Source: three-view drawing plus pictorial views. Frame: mm from the lowest corner of the part. A direction names the side the tool comes from. Give positions to 0.01 mm unless a question says otherwise; leave off trailing zeros. Loops run counter-clockwise (first coordinate to the right, second up) from the corner with the lowest first, then second, coordinate; pieces in that order, holes last. Notation, with made-up numbers: M -5,-6.75 L 33,-6.75 A12 cw 33,3.25 Z; hole C 30,71.25 d5. An arc over 180 degrees is marked long. Answer as a JSON object with one key per item and string values. Group by question number.
1) Ray query, L1, parallel to Y at x = 20, z = 12; L2, parallel to X at y = 20, z = 13; L3, parallel to X at y = 12, z = 13.5. Return the intervals inside material, ascending.
2) Access query for the marked faces 1 and 2. Directions: +Z, -Z, +X, -X, +Y, -Y. A direction counts if a zero-diameter tool reaches every point of the face in a straight line with its end or side. Return the directions, or none.
3) Draft query along Y for the marked faces 3, 4 and 5. Return one class per face: +Y half, -Y half, draft (parallel to the pull), parting line (faces both ways), or undercut.
4) Section query B-B on z = 12.5. Return loops of the section in (x, y), plus the area to 3 significant figures.
5) Section query D-D on x = 49. Return loops of the section in (y, z).
6) Section query A-A on x = 20. Return loops of the section in (y, z), plus the area to 3 significant figures.
7) First-contact query: P1, Ø5, axis at x = 4, z = 27, coming from the +Y side; P2, Ø1.5, axis at x = 32.5, z = 8.5, coming from the +Y side; P3, Ø6, axis at x = 36, y = 32, coming from the +Z side. Flat tips, straight axial feed; report the tip coordinate or a pass-through.
8) Section query C-C on y = 14.5. Return loops of the section in (x, z), plus the area to 3 significant figures.
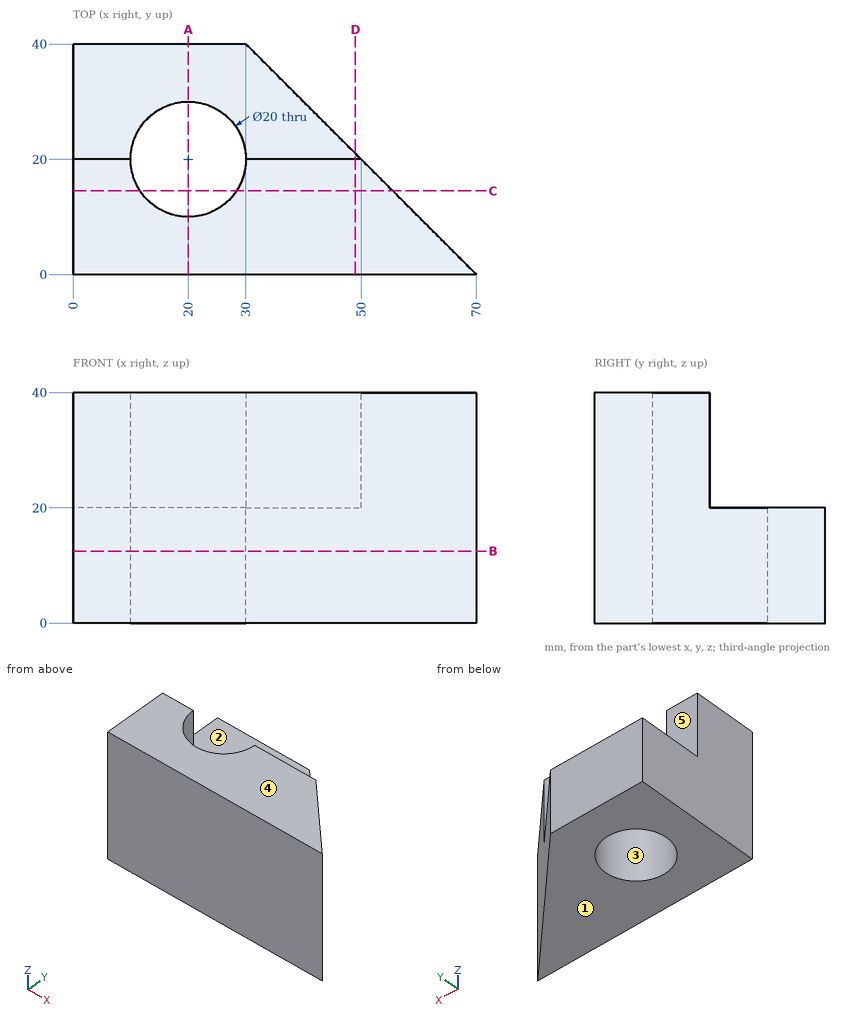
Output:
{
 "1": {"L1": "y = 0 to 10, 30 to 40", "L2": "x = 0 to 10, 30 to 50", "L3": "x = 0 to 14, 26 to 58"},
 "2": {"face 1": "-Z, +X, -X, +Y, -Y", "face 2": "+Z, +X, -X, +Y"},
 "3": {"face 3": "undercut", "face 4": "draft", "face 5": "+Y half"},
 "4": {"outline": "M 0,0 L 70,0 L 30,40 L 0,40 Z; hole C 20,20 d20", "area": "1,690 mm^2"},
 "5": {"outline": "M 0,0 L 21,0 L 21,20 L 20,20 L 20,40 L 0,40 Z"},
 "6": {"outline": "M 0,0 L 10,0 L 10,40 L 0,40 Z; M 30,0 L 40,0 L 40,20 L 30,20 Z", "area": "600 mm^2"},
 "7": {"P1": "stops at y = 20", "P2": "stops at y = 38.25", "P3": "stops at z = 20"},
 "8": {"outline": "M 0,0 L 11.65,0 L 11.65,40 L 0,40 Z; M 28.35,0 L 55.5,0 L 55.5,40 L 28.35,40 Z", "area": "1,550 mm^2"}
}
